For this review, take the finished solid that the model builds, in its own axes (mm). Give positions to 0.01 mm unless a question says otherwise; leave off trailing zeros. Loops run counter-clockwise (first coordinate to the right, second up) from the corner with the lowest first, then second, coordinate; pieces in that order, holes last.
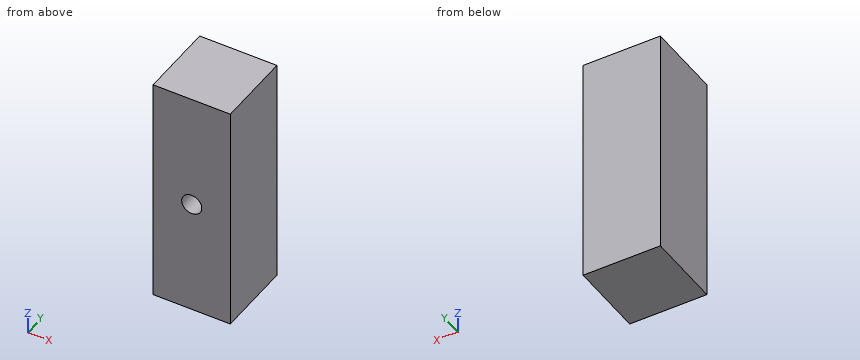
```python
from build123d import *

# Parameters (mm, degrees)
SKETCH1_W           = 20
SKETCH1_H           = 20
BOSS_EXTRUDE1_DEPTH = 60
SKETCH2_R           = 2.6
CUT_EXTRUDE1_DEPTH  = 5


with BuildPart() as part:
    # Sketch1 → Boss-Extrude1 (new body)
    with BuildSketch(Plane.XY):
        with Locations((10, -10)):
            Rectangle(SKETCH1_W, SKETCH1_H)
    extrude(amount=BOSS_EXTRUDE1_DEPTH)

    # Sketch2 → Cut-Extrude1 (cut)
    with BuildSketch(Plane.XZ.offset(20)):
        with Locations(Location((10, 30, 0), (0, 0, 270))):
            Circle(SKETCH2_R)
    extrude(amount=-CUT_EXTRUDE1_DEPTH, mode=Mode.SUBTRACT)


solid = part.part
```
Item 1: For L1, parallel to X at y = -16.45, z = 30; L2, parallel to Z at x = 9, y = -15.25, list the stretches that pass through material, from the lowest coordinate up.
Answer:
L1: x = 0 to 7.4, 12.6 to 20
L2: z = 0 to 27.6, 32.4 to 60
Item 2: Take a section at C-C on z = 30. Give the boundary of the cut face in (x, y), and give its area (3 significant figures).
Answer:
outline: (0, -20) - (7.4, -20) - (7.4, -15) - (12.6, -15) - (12.6, -20) - (20, -20) - (20, 0) - (0, 0) - close
area: 374 mm2
Item 3: Take a section at B-B on x = 10. Give the boundary of the cut face in (y, z).
Answer:
outline: (-20, 0) - (0, 0) - (0, 60) - (-20, 60) - (-20, 32.6) - (-15, 32.6) - (-15, 27.4) - (-20, 27.4) - close
Item 4: Clearance check with flat-ended pins moving along their axes: pin 1 Ø8.5 at (x, z) = (10, 30) entering from +Y; pin 2 Ø2.5 at (x, z) = (9, 29.5) entering from -Y. State where each tip first meets the part, or that it passes through.
Answer:
pin 1: stops at y = 0
pin 2: stops at y = -15
Item 5: Take a section at A-A on y = -17. Give the boundary of the cut face in (x, z), and give its area (3 significant figures).
Answer:
outline: (0, 0) - (20, 0) - (20, 60) - (0, 60) - close; hole circle Ø5.2 at (10, 30)
area: 1,180 mm2
